from build123d import *

# Parameters (mm, degrees)
SKETCH_1_R      = 2.001727574
SKETCH_1_R_2    = 1.895105282
EXTRUDE_1_DEPTH = 5.5
FILLET_1_R      = 3


with BuildPart() as part:
    # 草图1 → 凸台-拉伸1 (new body)
    with BuildSketch(Plane.XY):
        Polygon((-8, 15), (8, 15), (26, 15), (26, -5), (8, -5), (8, -15), (-8, -15), align=None)
        with Locations((-5, 10)):
            Circle(SKETCH_1_R, mode=Mode.SUBTRACT)
        with Locations((5, 10)):
            Circle(SKETCH_1_R, mode=Mode.SUBTRACT)
        with Locations((5, 0)):
            Circle(SKETCH_1_R, mode=Mode.SUBTRACT)
        with Locations((5, -10)):
            Circle(SKETCH_1_R, mode=Mode.SUBTRACT)
        with Locations((-5, 0)):
            Circle(SKETCH_1_R, mode=Mode.SUBTRACT)
        with Locations((-5, -10)):
            Circle(SKETCH_1_R, mode=Mode.SUBTRACT)
        with Locations((15, 10)):
            Circle(SKETCH_1_R_2, mode=Mode.SUBTRACT)
        with Locations((21, 10)):
            Circle(SKETCH_1_R_2, mode=Mode.SUBTRACT)
        with Locations((21, 0)):
            Circle(SKETCH_1_R_2, mode=Mode.SUBTRACT)
        with Locations((15, 0)):
            Circle(SKETCH_1_R_2, mode=Mode.SUBTRACT)
    extrude(amount=EXTRUDE_1_DEPTH)

    # 圆角1
    fillet_1_edges = [part.edges().sort_by_distance(p)[0] for p in [
        (8, -15, 2.75),
        (-8, -15, 2.75),
        (-8, 15, 2.75),
        (26, 15, 2.75),
        (26, -5, 2.75),
        (8, -5, 2.75),
    ]]
    fillet(fillet_1_edges, radius=FILLET_1_R)


solid = part.part
Input: part model. Units: mm. Frame: model coordinates. A direction names the side the tool comes from. Round coordinates to 2 decimals unless told otherwise and drop trailing zeros. Order: outer loops, then holes, each group sorted by start corner. A loop starts at its lowest first (then second) coordinate and runs counter-clockwise, first axis right, second up.
1. Material intervals for line 1 (Y direction, x = 21, z = 3.15); line 2 (Y direction, x = -5, z = 2.4); line 3 (X direction, y = 9, z = 0.55), sorted ascending.
The answers:
line 1: y = -5 to -1.9, 1.9 to 8.1, 11.9 to 15
line 2: y = -15 to -12, -8 to -2, 2 to 8, 12 to 15
line 3: x = -8 to -6.73, -3.27 to 3.27, 6.73 to 13.39, 16.61 to 19.39, 22.61 to 26
2. Mould query, pull axis Y, two halves, no side actions, for faces 1 (the face through (25.1, 14.14, 2.79)), 2 (the face through (3, 0, 3)), 3 (the face through (3.4, 8.8, 2.7)), 4 (the face through (8.9, -5.86, 2.79)). Classes: released by +Y, released by -Y, zero draft, split by the parting line, or undercut.
The answers:
face 1: released by +Y
face 2: undercut
face 3: undercut
face 4: released by -Y
3. Set-up query: faces 5 (the face through (17, -5, 3)), 6 (the face through (26, 5, 3)). Return all of +Z, -Z, +X, -X, +Y, -Y with unobstructed straight access to the full face (end or side cutting, diameter ignored); none if empty.
The answers:
face 5: +Z, -Z, +X, -Y
face 6: +Z, -Z, +X, +Y, -Y
4. Pin query (flat end, axial travel): P1, Ø4, axis at x = 3, y = 7, coming from the -Z side; P2, Ø1.6, axis at x = 16, z = 3.5, coming from the -Y side; P3, Ø2.5, axis at x = -5, y = 0, coming from the +Z side; P4, Ø2, axis at y = -9.5, z = 2, coming from the +X side. Return the tip coordinate at first contact, or that it passes through.
The answers:
P1: stops at z = 0
P2: stops at y = -5
P3: passes through
P4: stops at x = 8
5. Cut plane B-B, the plane z = 4.2. State how many separate pieces and enclosed holes the cut face has, then the cut area to 3 significant figures.
The answers:
separate pieces: 1
enclosed holes: 10
area: 712 mm2
6. Cut plane D-D, the plane y = -11.25. Output: boundary loops of the cut face in (x, z), then the cut area to 3 significant figures.
The answers:
outline: (-8, 0) - (-6.56, 0) - (-6.56, 5.5) - (-8, 5.5) - close; (-3.44, 0) - (3.44, 0) - (3.44, 5.5) - (-3.44, 5.5) - close; (6.56, 0) - (8, 0) - (8, 5.5) - (6.56, 5.5) - close
area: 53.6 mm2
7. Cut plane A-A, the plane x = 15. Output: boundary loops of the cut face in (y, z).
The answers:
outline: (-5, 0) - (-1.9, 0) - (-1.9, 5.5) - (-5, 5.5) - close; (1.9, 0) - (8.1, 0) - (8.1, 5.5) - (1.9, 5.5) - close; (11.9, 0) - (15, 0) - (15, 5.5) - (11.9, 5.5) - close
8. Cut plane C-C, the plane y = 10. Output: boundary loops of the cut face in (x, z), then the cut area to 3 significant figures.
The answers:
outline: (-8, 0) - (-7, 0) - (-7, 5.5) - (-8, 5.5) - close; (-3, 0) - (3, 0) - (3, 5.5) - (-3, 5.5) - close; (7, 0) - (13.1, 0) - (13.1, 5.5) - (7, 5.5) - close; (16.9, 0) - (19.1, 0) - (19.1, 5.5) - (16.9, 5.5) - close; (22.9, 0) - (26, 0) - (26, 5.5) - (22.9, 5.5) - close
area: 101 mm2
